Can you work these out from the model? Positions are in its coordinate system, mm. Face numbers are marked on the shaded views. A direction names the side the tool comes from. Round coordinates to 2 decimals unless told otherwise and drop trailing zeros. Order: outer loops, then holes, each group sorted by start corner. A loop starts at its lowest first (then second) coordinate and runs counter-clockwise, first axis right, second up. Notation, with made-up numbers: M 79,81.25 L 85,81.25 A10 cw 85,99.25 Z; hole C -21,61 d3. An arc over 180 degrees is marked long. Answer as a JSON object with one key per item and string values. Group by question number.
from build123d import *

# Parameters (mm, degrees)
F0_W          = 550
F0_H          = 550
F1_DEPTH      = 50
F0_W_2        = 50
F0_H_2        = 50
F2_DEPTH      = 50
F2_DEPTH_BACK = 400


with BuildPart() as f1:
    # F0 (on Top) → F1 (new body)
    with BuildSketch(Plane.XY):
        Rectangle(F0_W, F0_H)
        Polygon((222.5, 272.5), (272.5, 272.5), (272.5, 222.5), (272.5, -222.5), (272.5, -272.5), (222.5, -272.5), (-222.5, -272.5), (-272.5, -272.5), (-272.5, -222.5), (-272.5, 222.5), (-272.5, 272.5), (-222.5, 272.5), align=None, mode=Mode.SUBTRACT)
        Polygon((222.5, 222.5), (222.5, 272.5), (-222.5, 272.5), (-222.5, 222.5), (-272.5, 222.5), (-272.5, -222.5), (-222.5, -222.5), (-222.5, -272.5), (222.5, -272.5), (222.5, -222.5), (272.5, -222.5), (272.5, 222.5), align=None)
    extrude(amount=F1_DEPTH)

    # F0 (on Top) → F2 (join, two sides)
    with BuildSketch(Plane.XY) as f2_sk:
        with Locations((-247.5, -247.5)):
            Rectangle(F0_W_2, F0_H_2)
        with Locations((247.5, -247.5)):
            Rectangle(F0_W_2, F0_H_2)
        with Locations((247.5, 247.5)):
            Rectangle(F0_W_2, F0_H_2)
        with Locations((-247.5, 247.5)):
            Rectangle(F0_W_2, F0_H_2)
    extrude(amount=F2_DEPTH)
    extrude(f2_sk.sketch, amount=-F2_DEPTH_BACK)


solid = f1.part
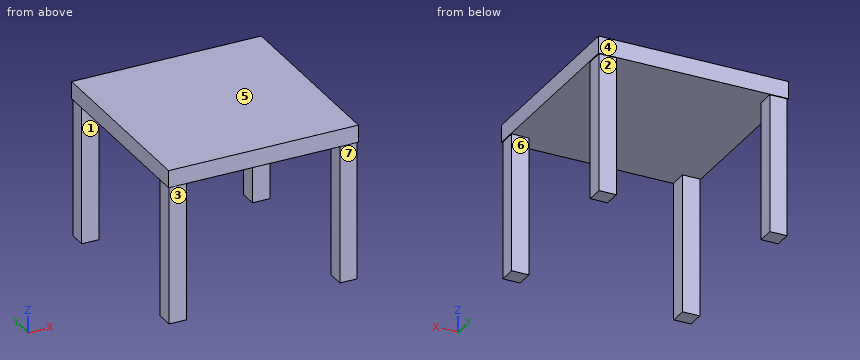
Item 1: If we mould it in two halves opening along Y, with no side actions, what happens to the marked faces 5, 6 and 7? For each: +Y half, -Y half, draft (parallel to the pull), parting line (faces both ways), or undercut.
Item 2: Suppose I cut it at C-C, the plane y = 117.5. Write out the boundary of the cut face in (x, z).
Item 3: Suppose I cut it at B-B, the plane x = -230. Write out the boundary of the cut face in (y, z).
Item 4: Suppose I cut it at A-A, the plane z = -64. Write out the boundary of the cut face in (x, y).
Item 5: On a 3-axis mill with a long thin cutter (end or side, diameter ignored), from which of +Z, -Z, +X, -X, +Y, -Y can I reach the whole of each face in a straight line? I mean the marked faces 1, 2, 3 and 4. Say none if no direction works.
Item 6: I need wall thicknesses on line 1 (X direction, y = 227.5, z = -374.5); line 2 (Z direction, x = -99, y = 232.5). Which ranges of each line are inside material? Lowest first, please.
Item 7: I'm going to push flat-ended pins straight in: pin 1 Ø15 at (x, z) = (255, -277) entering from +Y; pin 2 Ø25 at (y, z) = (243.5, -268.5) entering from -X; pin 3 Ø15 at (x, z) = (253.5, -227) entering from -Y. Where does each tip first touch, or does it pass through?
Computed:
{
 "1": {"face 5": "draft", "face 6": "undercut", "face 7": "-Y half"},
 "2": {"outline": "M -275,0 L 275,0 L 275,50 L -275,50 Z"},
 "3": {"outline": "M -275,0 L -272.5,0 L -272.5,-400 L -222.5,-400 L -222.5,0 L 222.5,0 L 222.5,-400 L 272.5,-400 L 272.5,0 L 275,0 L 275,50 L -275,50 Z"},
 "4": {"outline": "M -272.5,-272.5 L -222.5,-272.5 L -222.5,-222.5 L -272.5,-222.5 Z; M -272.5,222.5 L -222.5,222.5 L -222.5,272.5 L -272.5,272.5 Z; M 222.5,-272.5 L 272.5,-272.5 L 272.5,-222.5 L 222.5,-222.5 Z; M 222.5,222.5 L 272.5,222.5 L 272.5,272.5 L 222.5,272.5 Z"},
 "5": {"face 1": "-Z, +X, -X", "face 2": "-Z, +X, -X, +Y", "face 3": "-Z, +X, -X, -Y", "face 4": "+Z, -Z, +X, -X, +Y"},
 "6": {"line 1": "x = -272.5 to -222.5, 222.5 to 272.5", "line 2": "z = 0 to 50"},
 "7": {"pin 1": "stops at y = 272.5", "pin 2": "stops at x = -272.5", "pin 3": "stops at y = -272.5"}
}
